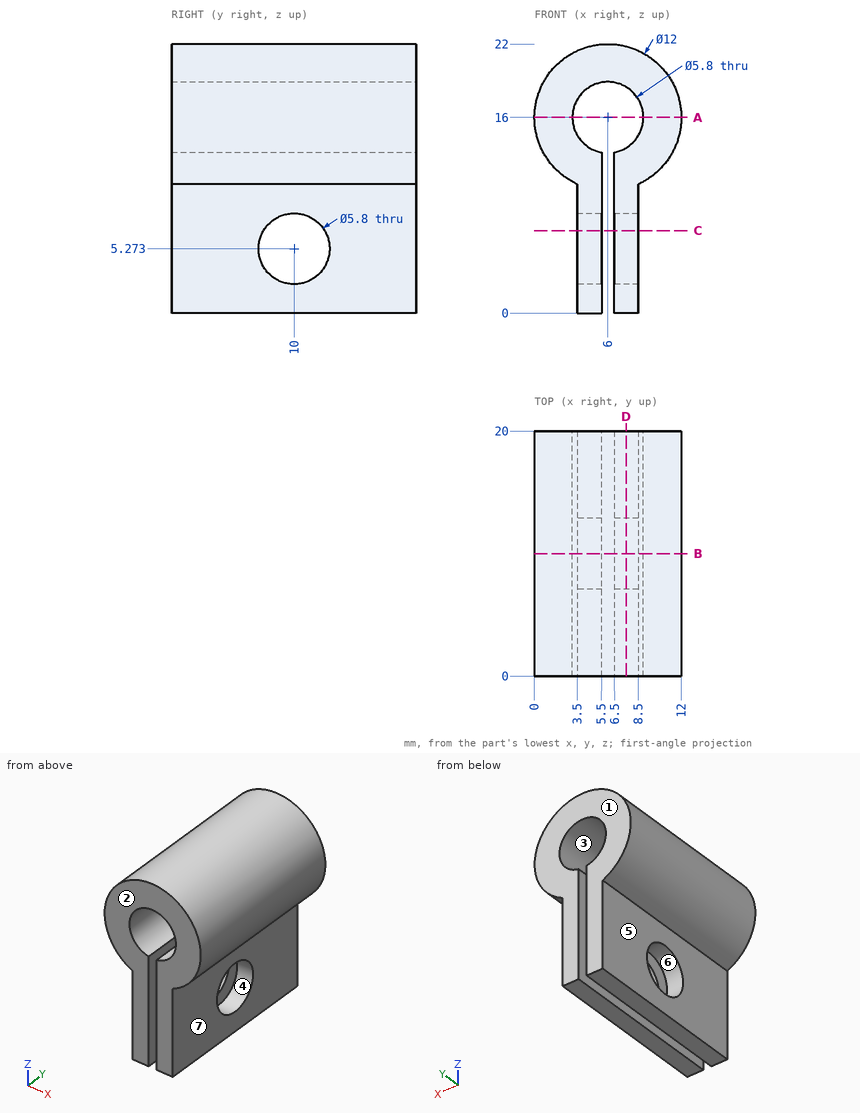
Geometry check sheet. Reference: drawing and pictorial views, mm from the part's lowest x, y, z. A direction names the side the tool comes from. Give positions to 0.01 mm unless a question says otherwise; leave off trailing zeros. Order: outer loops, then holes, each group sorted by start corner. A loop starts at its lowest first (then second) coordinate and runs counter-clockwise, first axis right, second up.
1. Section check C-C, the plane z = 6.75. Enter the section's corners in (x, y).
2. Access from +Z, -Z, +X, -X, +Y, -Y to the whole of each face (thin tool, end or side, straight path). Record for the marked faces 5, 6 and 7.
3. Thickness scan on L1, parallel to X at y = 14, z = 16; L2, parallel to X at y = 12, z = 9.5; L3, parallel to Z at x = 6, y = 14.5. Record the ranges inside material, lowest first.
4. Section check D-D, the plane x = 7.5. Enter the section's corners in (y, z).
5. Section check A-A, the plane z = 16. Enter the section's corners in (x, y).
6. Section check B-B, the plane y = 10. Enter the section's corners in (x, z), and give its area (3 significant figures).
7. Release check for a two-part mould opening along Y. For the marked faces 1, 2, 3 and 4 record: pulls with the +Y half, pulls with the -Y half, needs draft (parallel to the pull), parting line crosses it, or undercut.
8. Gauge pin test, flat ends, axial feed: pin 1 Ø5 at (y, z) = (10, 5.27) entering from +X (3 decimals); pin 2 Ø8.5 at (y, z) = (13.5, 4.5) entering from +X; pin 3 Ø8.5 at (y, z) = (10.5, 7.5) entering from -X (1 decimal); pin 4 Ø2 at (y, z) = (14, 18.5) entering from -X. Record the tip position at first contact, or that the pin passes through.
Values follow:
1. outline: (3.5, 0) - (5.5, 0) - (5.5, 7.5) - (3.5, 7.5) - close; (3.5, 12.5) - (5.5, 12.5) - (5.5, 20) - (3.5, 20) - close; (6.5, 0) - (8.5, 0) - (8.5, 7.5) - (6.5, 7.5) - close; (6.5, 12.5) - (8.5, 12.5) - (8.5, 20) - (6.5, 20) - close
2. face 5: -Z, -X, +Y, -Y
2. face 6: +X, -X
2. face 7: -Z, +X, +Y, -Y
3. L1: x = 0 to 3.1, 8.9 to 12
3. L2: x = 3.5 to 5.5, 6.5 to 8.5
3. L3: z = 18.9 to 22
4. outline: (0, 0) - (20, 0) - (20, 13.52) - (0, 13.52) - close; (0, 18.48) - (20, 18.48) - (20, 21.81) - (0, 21.81) - close; hole circle Ø5.8 at (10, 5.27)
5. outline: (0, 0) - (3.1, 0) - (3.1, 20) - (0, 20) - close; (8.9, 0) - (12, 0) - (12, 20) - (8.9, 20) - close
6. outline: (3.5, 0) - (5.5, 0) - (5.5, 2.37) - (3.5, 2.37) - close; (3.5, 8.17) - (5.5, 8.17) - (5.5, 13.14) arc R2.9 cw (long way) to (6.5, 13.14) - (6.5, 8.17) - (8.5, 8.17) - (8.5, 10.55) arc R6 ccw (long way) to (3.5, 10.55) - close; (6.5, 0) - (8.5, 0) - (8.5, 2.37) - (6.5, 2.37) - close
6. area: 101 mm2
7. face 1: pulls with the +Y half
7. face 2: pulls with the -Y half
7. face 3: needs draft
7. face 4: undercut
8. pin 1: passes through
8. pin 2: stops at x = 8.5
8. pin 3: stops at x = 1.8
8. pin 4: stops at x = 0.19
